Geometry: final body of the model. Coordinates: model frame, mm. A direction names the side the tool comes from. Give positions to 0.01 mm unless a question says otherwise; leave off trailing zeros. Order: outer loops, then holes, each group sorted by start corner. A loop starts at its lowest first (then second) coordinate and runs counter-clockwise, first axis right, second up. Notation, with made-up numbers: (87, -29.5) -> (125, -29.5) arc R23 ccw to (125, -2.5) -> close; hole circle Ø10 at (36.25, 82). An arc over 180 degrees is marked (long way). One line per question, with ' | ' between items.
from build123d import *

# Parameters (mm, degrees)
SKETCH1_R               = 31.75
SKETCH1_R_2             = 2.7
SKETCH1_R_3             = 2.6999999999999793
SKETCH1_R_4             = 2.699999999999988
SKETCH1_R_5             = 2.7000000000000046
BOSS_EXTRUDE1_DEPTH     = 4
SKETCH2_R               = 4.000000000000011
SKETCH2_R_2             = 2.7
BOSS_EXTRUDE2_DEPTH     = 28.823381129999998
SKETCH3_R               = 5.000000000000011
SKETCH3_R_2             = 4.000000000000011
BOSS_EXTRUDE3_DEPTH     = 1.5
BOSS_EXTRUDE4_DEPTH     = 28.823381129999998
FILLET2_R               = 0.5
FILLET5_R               = 1.61977879287575
CIRPATTERN1_START       = 4
CIRPATTERN1_DEPTH       = 28.82338113
CHAMFER1_SIZE           = 0.5
SKETCH9_R               = 8
CUT_EXTRUDE4_DEPTH      = 54.35646463391214
BOSS_EXTRUDE7_START     = -6.5
SKETCH10_R              = 8
SKETCH10_R_2            = 6.500000000000002
BOSS_EXTRUDE7_DEPTH     = 6.5
CUT_EXTRUDE5_DEPTH      = 54.35646463391214
CUT_EXTRUDE5_DEPTH_BACK = 54.35646463391214
SKETCH14_R              = 16.1
SKETCH15_R              = 16.1
SKETCH15_R_2            = 15.1
BOSS_EXTRUDE8_DEPTH     = 1.5
SKETCH16_R              = 18.099999999999998
SKETCH16_R_2            = 16.1
BOSS_EXTRUDE9_DEPTH     = 4.5
CHAMFER3_SIZE2          = 4.5
CHAMFER3_SIZE           = 2
SKETCH5_R               = 1.6999999999999995
CUT_EXTRUDE1_DEPTH      = 59.38801068434546
CUT_EXTRUDE3_START      = -5
SKETCH7_R               = 4.45
CUT_EXTRUDE3_DEPTH      = 61.61923559408127
CUT_EXTRUDE2_START      = -3
SKETCH6_R               = 2.949999999999982
CUT_EXTRUDE2_DEPTH      = 59.61923559408127
CIRPATTERN2_COUNT       = 4
CHAMFER4_SIZE           = 0.5


# Read off the part's stored shape, not the designer's step: CirPattern1
with BuildPart() as part:
    # Sketch1 → Boss-Extrude1 (new body)
    with BuildSketch(Plane.XY):
        Circle(SKETCH1_R)
        with Locations((0, 26)):
            Circle(SKETCH1_R_2, mode=Mode.SUBTRACT)
        with Locations((26, 1.59e-15)):
            Circle(SKETCH1_R_3, mode=Mode.SUBTRACT)
        with Locations((3.18e-15, -26)):
            Circle(SKETCH1_R_4, mode=Mode.SUBTRACT)
        with Locations((-26, 1.59e-15)):
            Circle(SKETCH1_R_5, mode=Mode.SUBTRACT)
    extrude(amount=BOSS_EXTRUDE1_DEPTH)

    # Sketch2 → Boss-Extrude2 (add)
    with BuildSketch(Plane.XY.offset(4)):
        with Locations((0, 26)):
            Circle(SKETCH2_R)
        with Locations((0, 26)):
            Circle(SKETCH2_R_2, mode=Mode.SUBTRACT)
    extrude(amount=BOSS_EXTRUDE2_DEPTH)

    # Sketch3 → Boss-Extrude3 (add)
    with BuildSketch(Plane.XY.offset(4)):
        with Locations((0, 26)):
            Circle(SKETCH3_R)
        with Locations((0, 26)):
            Circle(SKETCH3_R_2, mode=Mode.SUBTRACT)
    extrude(amount=BOSS_EXTRUDE3_DEPTH)

    # Sketch4 → Boss-Extrude4 (add)
    with BuildSketch(Plane.XY.offset(4)):
        with BuildLine():
            ThreePointArc((-9.529354319679797, 16.437499999999996), (-12.951492793939106, 22.190953609032412), (-13.189002373040246, 28.881009615384613))
            ThreePointArc((-13.189002373040248, 28.881009615384617), (-22.45064030267292, 22.450640302672845), (-28.88100961538466, 13.189002373040152))
            ThreePointArc((-28.88100961538466, 13.18900237304014), (-22.19095360903246, 12.951492793939027), (-16.437500000000036, 9.529354319679738))
            ThreePointArc((-16.437500000000036, 9.529354319679735), (-13.435028842544424, 13.43502884254438), (-9.529354319679797, 16.4375))
        make_face()
    extrude(amount=BOSS_EXTRUDE4_DEPTH)

    # Fillet2
    fillet2_edges = [part.edges().sort_by_distance(p)[0] for p in [
        (-5.000000000000011, 26, 5.5),
    ]]
    fillet(fillet2_edges, radius=FILLET2_R)

    # Fillet5
    fillet5_edges = [part.edges().sort_by_distance(p)[0] for p in [
        (-13.189002373040246, 28.881009615384613, 18.411690565),
        (-28.881009615384663, 13.189002373040147, 18.411690565),
        (-16.437500000000036, 9.529354319679737, 18.411690565),
        (-9.529354319679797, 16.4375, 18.411690565),
    ]]
    fillet(fillet5_edges, radius=FILLET5_R)

    # CirPattern1 outline → CirPattern1 (add)
    with BuildSketch(Plane.XY.offset(CIRPATTERN1_START)):
        with BuildLine():
            ThreePointArc((-15.461987637, -11.042053175), (-16.542214144, -10.381196466), (-17.767866629, -10.699625235))
            ThreePointArc((-17.767866629, -10.699625235), (-21.67849749, -12.789629238), (-26.055332527, -13.499886604))
            ThreePointArc((-26.055332527, -13.499886604), (-27.463927582, -14.308354959), (-27.463044171, -15.932473282))
            ThreePointArc((-27.463044171, -15.932473282), (-22.450640303, -22.450640303), (-15.932473282, -27.463044171))
            ThreePointArc((-15.932473282, -27.463044171), (-14.308354959, -27.463927582), (-13.499886604, -26.055332527))
            ThreePointArc((-13.499886604, -26.055332527), (-12.789629238, -21.67849749), (-10.699625235, -17.767866629))
            ThreePointArc((-10.699625235, -17.767866629), (-10.381196466, -16.542214144), (-11.042053175, -15.461987637))
            ThreePointArc((-11.042053175, -15.461987637), (-13.435028843, -13.435028843), (-15.461987637, -11.042053175))
        make_face()
        with BuildLine():
            ThreePointArc((27.463044171, 15.932473282), (22.450640303, 22.450640303), (15.932473282, 27.463044171))
            ThreePointArc((15.932473282, 27.463044171), (14.308354959, 27.463927582), (13.499886604, 26.055332527))
            ThreePointArc((13.499886604, 26.055332527), (12.789629238, 21.67849749), (10.699625235, 17.767866629))
            ThreePointArc((10.699625235, 17.767866629), (10.381196466, 16.542214144), (11.042053175, 15.461987637))
            ThreePointArc((11.042053175, 15.461987637), (13.435028843, 13.435028843), (15.461987637, 11.042053175))
            ThreePointArc((15.461987637, 11.042053175), (16.542214144, 10.381196466), (17.767866629, 10.699625235))
            ThreePointArc((17.767866629, 10.699625235), (21.67849749, 12.789629238), (26.055332527, 13.499886604))
            ThreePointArc((26.055332527, 13.499886604), (27.463927582, 14.308354959), (27.463044171, 15.932473282))
        make_face()
        with BuildLine():
            ThreePointArc((13.499886604, -26.055332527), (14.308354959, -27.463927582), (15.932473282, -27.463044171))
            ThreePointArc((15.932473282, -27.463044171), (22.450640303, -22.450640303), (27.463044171, -15.932473282))
            ThreePointArc((27.463044171, -15.932473282), (27.463927582, -14.308354959), (26.055332527, -13.499886604))
            ThreePointArc((26.055332527, -13.499886604), (21.67849749, -12.789629238), (17.767866629, -10.699625235))
            ThreePointArc((17.767866629, -10.699625235), (16.542214144, -10.381196466), (15.461987637, -11.042053175))
            ThreePointArc((15.461987637, -11.042053175), (13.435028843, -13.435028843), (11.042053175, -15.461987637))
            ThreePointArc((11.042053175, -15.461987637), (10.381196466, -16.542214144), (10.699625235, -17.767866629))
            ThreePointArc((10.699625235, -17.767866629), (12.789629238, -21.67849749), (13.499886604, -26.055332527))
        make_face()
    extrude(amount=CIRPATTERN1_DEPTH)

    # CirPattern1 2 outline → CirPattern1 2 (revolve)
    with BuildSketch(Plane(origin=(-26, 0, 0), x_dir=(1, 0, 0), z_dir=(0, -1, 0))):
        with BuildLine():
            Line((4, 32.82338113), (2.7, 32.82338113))
            Line((2.7, 32.82338113), (2.7, 4))
            Line((2.7, 4), (5, 4))
            Line((5, 4), (5, 5))
            ThreePointArc((5, 5), (4.853553391, 5.353553391), (4.5, 5.5))
            Line((4.5, 5.5), (4, 5.5))
            Line((4, 5.5), (4, 32.82338113))
        make_face()
    revolve(axis=Axis((-26, 0, 0), (0, 0, 1)))

    # CirPattern1 3 outline → CirPattern1 3 (revolve)
    with BuildSketch(Plane.XZ.offset(26)):
        with BuildLine():
            Line((4, 32.82338113), (2.7, 32.82338113))
            Line((2.7, 32.82338113), (2.7, 4))
            Line((2.7, 4), (5, 4))
            Line((5, 4), (5, 5))
            ThreePointArc((5, 5), (4.853553391, 5.353553391), (4.5, 5.5))
            Line((4.5, 5.5), (4, 5.5))
            Line((4, 5.5), (4, 32.82338113))
        make_face()
    revolve(axis=Axis((0, -26, 0), (0, 0, 1)))

    # CirPattern1 4 outline → CirPattern1 4 (revolve)
    with BuildSketch(Plane(origin=(26, 0, 0), x_dir=(1, 0, 0), z_dir=(0, -1, 0))):
        with BuildLine():
            Line((4, 32.82338113), (2.7, 32.82338113))
            Line((2.7, 32.82338113), (2.7, 4))
            Line((2.7, 4), (5, 4))
            Line((5, 4), (5, 5))
            ThreePointArc((5, 5), (4.853553391, 5.353553391), (4.5, 5.5))
            Line((4.5, 5.5), (4, 5.5))
            Line((4, 5.5), (4, 32.82338113))
        make_face()
    revolve(axis=Axis((26, 0, 0), (0, 0, 1)))

    # Chamfer1
    chamfer1_edges = [part.edges().sort_by_distance(p)[0] for p in [
        (-31.75, 3.89e-15, 0),
    ]]
    chamfer(chamfer1_edges, length=CHAMFER1_SIZE)

    # Sketch9 → Cut-Extrude4 (cut, through all)
    with BuildSketch(Plane.XY.offset(4)):
        Circle(SKETCH9_R)
    extrude(amount=-CUT_EXTRUDE4_DEPTH, mode=Mode.SUBTRACT)

    # Sketch10 → Boss-Extrude7 (add)
    with BuildSketch(Plane(origin=(0, 0, 0), x_dir=(-1, 0, 0), z_dir=(0, 0, -1)).offset(BOSS_EXTRUDE7_START)):
        Circle(SKETCH10_R)
        Circle(SKETCH10_R_2, mode=Mode.SUBTRACT)
    extrude(amount=BOSS_EXTRUDE7_DEPTH)

    # Sketch14 → Cut-Extrude5 (cut, two sides: drawn at the far end of the back side and taken through both)
    with BuildSketch(Plane.XY.offset(4).offset(-CUT_EXTRUDE5_DEPTH_BACK)):
        Circle(SKETCH14_R)
    extrude(amount=CUT_EXTRUDE5_DEPTH + CUT_EXTRUDE5_DEPTH_BACK, mode=Mode.SUBTRACT)

    # Sketch15 → Boss-Extrude8 (add)
    with BuildSketch(Plane.XY.offset(4)):
        Circle(SKETCH15_R)
        Circle(SKETCH15_R_2, mode=Mode.SUBTRACT)
    extrude(amount=-BOSS_EXTRUDE8_DEPTH)

    # Sketch16 → Boss-Extrude9 (add)
    with BuildSketch(Plane(origin=(0, 0, 0), x_dir=(-1, 0, 0), z_dir=(0, 0, -1))):
        with Locations(Location((0, 0, 0), (0, 0, 180))):
            Circle(SKETCH16_R)
        with Locations(Location((0, 0, 0), (0, 0, 180))):
            Circle(SKETCH16_R_2, mode=Mode.SUBTRACT)
    extrude(amount=BOSS_EXTRUDE9_DEPTH)

    # Chamfer3
    chamfer3_edges = [part.edges().sort_by_distance(p)[0] for p in [
        (-18.099999999999998, -4.43e-15, 0),
    ]]
    chamfer3_side = [part.faces().sort_by_distance(p)[0] for p in [
        (-18.139999999999997, -4.44e-15, 0),
    ]]
    chamfer(chamfer3_edges, length=CHAMFER3_SIZE - 0.0001, length2=CHAMFER3_SIZE2 - 0.0001, reference=chamfer3_side[0])  # a hair under: the kernel refuses the full size

    # Sketch5 → Cut-Extrude1 (cut, through all)
    with BuildSketch(Plane.XY.offset(32.823381129999994)):
        with Locations((-19.622213177926728, 19.622213177926657)):
            Circle(SKETCH5_R)
    cut_extrude1 = extrude(amount=-CUT_EXTRUDE1_DEPTH, mode=Mode.SUBTRACT)

    # Sketch7 → Cut-Extrude3 (cut)
    with BuildSketch(Plane(origin=(0, 0, 0), x_dir=(-1, 0, 0), z_dir=(0, 0, -1)).offset(CUT_EXTRUDE3_START)):
        with Locations(Location((0, 26, 0), (0, 0, 180))):
            Circle(SKETCH7_R)
    cut_extrude3 = extrude(amount=CUT_EXTRUDE3_DEPTH, mode=Mode.SUBTRACT)

    # Sketch6 → Cut-Extrude2 (cut)
    with BuildSketch(Plane(origin=(0, 0, 0), x_dir=(-1, 0, 0), z_dir=(0, 0, -1)).offset(CUT_EXTRUDE2_START)):
        with Locations(Location((19.622213177926728, 19.622213177926657, 0), (0, 0, 180))):
            Circle(SKETCH6_R)
    cut_extrude2 = extrude(amount=CUT_EXTRUDE2_DEPTH, mode=Mode.SUBTRACT)

    # CirPattern2: Cut-Extrude1, Cut-Extrude3, Cut-Extrude2 ×4 about axis
    cirpattern2_axis = Axis((-3.768e-14, -2.255e-14, 0), (0, 0, 1))
    add([cut_extrude1.rotate(cirpattern2_axis, i * 360 / CIRPATTERN2_COUNT) for i in range(1, CIRPATTERN2_COUNT)], mode=Mode.SUBTRACT)
    add([cut_extrude3.rotate(cirpattern2_axis, i * 360 / CIRPATTERN2_COUNT) for i in range(1, CIRPATTERN2_COUNT)], mode=Mode.SUBTRACT)
    add([cut_extrude2.rotate(cirpattern2_axis, i * 360 / CIRPATTERN2_COUNT) for i in range(1, CIRPATTERN2_COUNT)], mode=Mode.SUBTRACT)

    # Chamfer4
    chamfer4_edges = [part.edges().sort_by_distance(p)[0] for p in [
        (-16.1, -3.94e-15, -4.5),
    ]]
    chamfer(chamfer4_edges, length=CHAMFER4_SIZE)


solid = part.part
1) Section D-D on z = -1.5. Return loops of the section in (x, y).
Check result:
outline: circle Ø38.87 at (0, 0); hole circle Ø32.2 at (0, 0)
2) Section A-A on x = 0. Count the separate pieces of the cut face and the enclosed holes in it, plus the area to 3 significant figures.
Check result:
separate pieces: 4 | enclosed holes: 0 | area: 232 mm^2
3) Set-up query: faces 3 (the cylindrical face through (23.3, 0.1, 18.7)), 4 (the cylindrical face through (-30.995, 0.22, 4.507)), 5 (the cylindrical face through (16.697, 20.006, 1.521)). Return all of +Z, -Z, +X, -X, +Y, -Y with unobstructed straight access to the full face (end or side cutting, diameter ignored); none if empty.
Check result:
face 3: +Z, -Z | face 4: +Z | face 5: -Z
4) Pull-direction query (Y, two-part tool) for faces 1 (the cylindrical face through (-21.42, -21.96, 1.52)), 2 (the flat face through (19, 17, 32.823)); classes: +Y half, -Y half, draft (parallel to the pull), parting line (faces both ways), or undercut.
Check result:
face 1: undercut | face 2: draft
5) Contact query for flat-ended pins moving along their axis: pin 1 Ø7 at (x, y) = (-27, 1.5) entering from -Z; pin 2 Ø12 at (x, z) = (11.5, 13) entering from -Y; pin 3 Ø3 at (y, z) = (24, 9) entering from +X. Output: stop coordinate, or through.
Check result:
pin 1: stops at z = 0 | pin 2: stops at y = -27.68 | pin 3: stops at x = 22.4
6) Material intervals for probe 1 along Y at (x, z) = (0, 1.1); probe 2 along Y at (x, z) = (-21, 25); probe 3 along X at (y, z) = (-20, 29), sorted ascending. Write a range as from..to.
Check result:
probe 1: y = -31.75..-30.45, -21.55..-16.1, 16.1..21.55, 30.45..31.75 | probe 2: y = -23.81..-20.62, -18.63..-12.54, 12.54..18.63, 20.62..23.81 | probe 3: x = -24.66..-21.28, -17.96..-12.09, 12.09..17.96, 21.28..24.66
